Could you check a few things on this model? Use its own coordinates, in mm. A direction names the side the tool comes from. Round coordinates to 2 decimals unless told otherwise and drop trailing zeros. Loops run counter-clockwise (first coordinate to the right, second up) from the corner with the lowest first, then second, coordinate; pieces in that order, holes last. Notation, with made-up numbers: M -8.75,85 L 18.25,85 A30 ccw 18.25,121 Z; hole C 36,79 d9. An arc over 180 degrees is marked long. Return JSON: item names as keys, results as strings. Group by question number.
```python
from build123d import *

# Parameters (mm, degrees)
SKETCH1_R               = 7.62
SKETCH1_R_2             = 6.35
BOSS_EXTRUDE1_DEPTH     = 165.1
CUT_EXTRUDE1_REACH      = 167.977
CUT_EXTRUDE1_END_RADIUS = 6.35
FILLET3_R               = 2.54


with BuildPart() as part:
    # Sketch1 → Boss-Extrude1 (new body)
    with BuildSketch(Plane(origin=(0, 0, 0), x_dir=(1, 0, 0), z_dir=(0, 1, 0))):
        with Locations(Location((0, 0, 0), (0, 0, 270))):
            Circle(SKETCH1_R)
        with Locations(Location((0, 0, 0), (0, 0, 270))):
            Circle(SKETCH1_R_2, mode=Mode.SUBTRACT)
    extrude(amount=BOSS_EXTRUDE1_DEPTH)

    # Cut-Extrude1: up to this cylinder (the profile starts outside it)
    cut_extrude1_end = Plane(origin=(0, 137.302889, 0), z_dir=(0, -1, 0)) * Cylinder(CUT_EXTRUDE1_END_RADIUS, 360.824706, mode=Mode.PRIVATE)
    # Sketch2 → Cut-Extrude1 (cut, up to the surface)
    with BuildSketch(Plane.ZY.offset(7.62), mode=Mode.PRIVATE) as cut_extrude1_sk1:
        with BuildLine():
            Line((-2.286, 154.058948498), (-2.286, 131.717535749))
            ThreePointArc((-2.286, 131.717535749), (-3.81, 130.193535749), (-5.334, 131.717535749))
            Line((-5.334, 131.717535749), (-5.334, 154.058948498))
            ThreePointArc((-5.334, 154.058948498), (-3.81, 155.582948498), (-2.286, 154.058948498))
        make_face()
    cut_extrude1_tool1 = extrude(cut_extrude1_sk1.sketch, amount=-CUT_EXTRUDE1_REACH, mode=Mode.PRIVATE) - cut_extrude1_end
    add(cut_extrude1_tool1.solids().sort_by_distance((-7.62, 142.888242, -3.81))[0], mode=Mode.SUBTRACT)
    # Sketch2 → Cut-Extrude1 (cut, up to the surface)
    with BuildSketch(Plane.ZY.offset(7.62), mode=Mode.PRIVATE) as cut_extrude1_sk2:
        with BuildLine():
            Line((2.286, 131.717535749), (2.286, 138.086901397))
            ThreePointArc((2.286, 138.086901397), (3.81, 139.610901397), (5.334, 138.086901397))
            Line((5.334, 138.086901397), (5.334, 131.717535749))
            ThreePointArc((5.334, 131.717535749), (3.81, 130.193535749), (2.286, 131.717535749))
        make_face()
    cut_extrude1_tool2 = extrude(cut_extrude1_sk2.sketch, amount=-CUT_EXTRUDE1_REACH, mode=Mode.PRIVATE) - cut_extrude1_end
    add(cut_extrude1_tool2.solids().sort_by_distance((-7.62, 134.902219, 3.81))[0], mode=Mode.SUBTRACT)
    # Sketch2 → Cut-Extrude1 (cut, up to the surface)
    with BuildSketch(Plane.ZY.offset(7.62), mode=Mode.PRIVATE) as cut_extrude1_sk3:
        with BuildLine():
            Line((-3.81, 133.241535749), (3.81, 133.241535749))
            ThreePointArc((3.81, 133.241535749), (5.334, 131.717535749), (3.81, 130.193535749))
            Line((3.81, 130.193535749), (-3.81, 130.193535749))
            ThreePointArc((-3.81, 130.193535749), (-5.334, 131.717535749), (-3.81, 133.241535749))
        make_face()
    cut_extrude1_tool3 = extrude(cut_extrude1_sk3.sketch, amount=-CUT_EXTRUDE1_REACH, mode=Mode.PRIVATE) - cut_extrude1_end
    add(cut_extrude1_tool3.solids().sort_by_distance((-7.62, 131.717536, 0))[0], mode=Mode.SUBTRACT)

    # Fillet3
    # the kernel refuses this fillet: 2.54 mm, written as the material it takes off along each edge
    with BuildSketch(Plane(origin=(-13.619016715, 133.241535749, 2.286), x_dir=(0, 0, -1), z_dir=(1, 0, 0)), Plane(origin=(0.425752875, 133.241535749, -2.286), x_dir=(0, 0, 1), z_dir=(-1, 0, 0))) as fillet3_piece_1:
        with BuildLine():
            CenterArc((FILLET3_R, FILLET3_R), FILLET3_R, 180, 90)
            Line((0, FILLET3_R), (0, 0))
            Line((0, 0), (FILLET3_R, 0))
        make_face()
    extrude(amount=14.04476959, mode=Mode.SUBTRACT)


solid = part.part
```
1. I'm going to push flat-ended pins straight in: pin 1 Ø1.1 at (x, y) = (-6.5, 136.5) entering from +Z; pin 2 Ø8 at (x, z) = (-2.5, -5.5) entering from -Y; pin 3 Ø2 at (y, z) = (118, -5) entering from -X; pin 4 Ø1 at (y, z) = (89.5, 2.5) entering from +X. Where does each tip first touch, or does it pass through?
2. If we section it at B-B, the plane y = 67.5: Please give me the cut outline in (x, z), then the cut area to 3 significant figures.
3. We'd pull the mould along Z, two halves only. Please class faces 3 (the face through (-5.81, 139.61, 3.78)), 4 (the face through (-5.81, 155.48, -4.36)), 5 (the face through (7.555, 81.394, -0.992)), 6 (the face through (6, 165.1, -3)): +Z half, -Z half, draft (parallel to the pull), parting line (faces both ways), or undercut.
4. I need wall thicknesses on probe 1 along Z at (x, y) = (-0.5, 50); probe 2 along X at (y, z) = (122, 0); probe 3 along X at (y, z) = (84, -5.25). Which ranges of each line are inside material? Lowest first, please.
5. On a 3-axis mill with a long thin cutter (end or side, diameter ignored), from which of +Z, -Z, +X, -X, +Y, -Y can I reach the whole of each face in a straight line? I mean faces 1 (the face through (-7, 130.194, 0)), 2 (the face through (6, 0, -3)). Say none if no direction works.
6. If we section it at A-A, the plane x = 0: Please give me the cut outline in (y, z), then the cut area to 3 significant figures.
Geometry results:
{
 "1": {"pin 1": "z = 2.29", "pin 2": "y = 0", "pin 3": "x = -6.49", "pin 4": "x = 7.35"},
 "2": {"outline": "C 0,0 d15.24; hole C 0,0 d12.7", "area": "55.7 mm^2"},
 "3": {"face 3": "undercut", "face 4": "undercut", "face 5": "parting line", "face 6": "draft"},
 "4": {"probe 1": "-7.6 to -6.33, 6.33 to 7.6", "probe 2": "-7.62 to -6.35, 6.35 to 7.62", "probe 3": "-5.52 to -3.57, 3.57 to 5.52"},
 "5": {"face 1": "-X", "face 2": "+Z, -Z, +X, -X, -Y"},
 "6": {"outline": "M 0,-7.62 L 165.1,-7.62 L 165.1,-6.35 L 0,-6.35 Z; M 0,6.35 L 165.1,6.35 L 165.1,7.62 L 0,7.62 Z", "area": "419 mm^2"}
}
